```python
from build123d import *

# Parameters (mm, degrees)
SKETCH_W  = 7
SKETCH_H  = 29
SKETCH_R  = 1.65
PAD_DEPTH = 1.6
FILLET_R  = 2


with BuildPart() as part:
    # Sketch → Pad (new body)
    with BuildSketch(Plane.XY):
        with Locations((0, -9.5)):
            Rectangle(SKETCH_W, SKETCH_H)
        Circle(SKETCH_R, mode=Mode.SUBTRACT)
        with Locations((0, -10)):
            Circle(SKETCH_R, mode=Mode.SUBTRACT)
        with Locations((0, -20)):
            Circle(SKETCH_R, mode=Mode.SUBTRACT)
    extrude(amount=PAD_DEPTH)

    # Fillet
    fillet_edges = [part.edges().sort_by_distance(p)[0] for p in [
        (3.5, 5, 0.8),
        (3.5, -24, 0.8),
        (-3.5, -24, 0.8),
        (-3.5, 5, 0.8),
    ]]
    fillet(fillet_edges, radius=FILLET_R)


solid = part.part
```
Verification items for the finished model (mm, model axes). Coordinates: 2 decimals unless noted, no trailing zeros. Loops run counter-clockwise (first coordinate to the right, second up) from the corner with the lowest first, then second, coordinate; pieces in that order, holes last. Notation, with made-up numbers: (-13.75, -35.5) - (31.25, -35.5) arc R16 cw to (31.25, -12.5) - close; hole circle Ø7 at (35, 83). An arc over 180 degrees is marked (long way). Put each result on its own line as item: value.
Item 1: Section check D-D (x = 3.25). Enter the section's corners in (y, z).
Conclusion:
outline: (-22.97, 0) - (3.97, 0) - (3.97, 1.6) - (-22.97, 1.6) - close
Item 2: Section check C-C (z = 0.3). Enter the section's corners in (x, y), then the cut area to 3 significant figures.
Conclusion:
outline: (-3.5, -22) arc R2 ccw to (-1.5, -24) - (1.5, -24) arc R2 ccw to (3.5, -22) - (3.5, 3) arc R2 ccw to (1.5, 5) - (-1.5, 5) arc R2 ccw to (-3.5, 3) - close; hole circle Ø3.3 at (0, -20); hole circle Ø3.3 at (0, -10); hole circle Ø3.3 at (0, 0)
area: 174 mm2
Item 3: Section check B-B (x = 0). Enter the section's corners in (y, z), then the cut area to 3 significant figures.
Conclusion:
outline: (-24, 0) - (-21.65, 0) - (-21.65, 1.6) - (-24, 1.6) - close; (-18.35, 0) - (-11.65, 0) - (-11.65, 1.6) - (-18.35, 1.6) - close; (-8.35, 0) - (-1.65, 0) - (-1.65, 1.6) - (-8.35, 1.6) - close; (1.65, 0) - (5, 0) - (5, 1.6) - (1.65, 1.6) - close
area: 30.6 mm2
Item 4: Draft check along Y on faces 1 (the face through (-1.216, 1.115, 0.789)), 2 (the face through (-2.93, -23.4, 0.81)), 3 (the face through (0, 5, 1)). Enter one of: pulls with the +Y half, pulls with the -Y half, needs draft (parallel to the pull), parting line crosses it, or undercut.
Conclusion:
face 1: undercut
face 2: pulls with the -Y half
face 3: pulls with the +Y half
Item 5: Scan lines: line 1 along Y through (x, z) = (0, 1.2); line 2 along Y through (x, z) = (1, 1.15); line 3 along X through (y, z) = (-11.25, 1.05). Record each from-to range of solid material in increasing order.
Conclusion:
line 1: y = -24 to -21.65, -18.35 to -11.65, -8.35 to -1.65, 1.65 to 5
line 2: y = -24 to -21.31, -18.69 to -11.31, -8.69 to -1.31, 1.31 to 5
line 3: x = -3.5 to -1.08, 1.08 to 3.5
Item 6: Section check A-A (y = 0). Enter the section's corners in (x, z), then the cut area to 3 significant figures.
Conclusion:
outline: (-3.5, 0) - (-1.65, 0) - (-1.65, 1.6) - (-3.5, 1.6) - close; (1.65, 0) - (3.5, 0) - (3.5, 1.6) - (1.65, 1.6) - close
area: 5.92 mm2
